from build123d import *

# Parameters (mm, degrees)
F3_W           = 38.1
F3_H           = 32.95
F3_W_2         = 34.5
F3_H_2         = 29.35
F4_DEPTH       = 102
F6_W           = 5.6
F6_H           = 6
F7_DEPTH       = 1.8
F5_R           = 1.5
F9_DEPTH       = 2
F10_DEPTH      = 32.951
F10_DEPTH_BACK = 25
F11_W          = 38.1
F11_H          = 34.95
F12_DEPTH      = 1.8
F14_DEPTH      = 3.8
F15_R          = 2.7
F16_DEPTH      = 2
F16_DEPTH_BACK = 31.151
F17_DEPTH      = 31.15
F19_DEPTH      = 25
F20_R          = 2.5
F21_R          = 2
F24_DEPTH      = 28
F25_R          = 0.89999


# Not quite as in the source:
# - a fillet or chamfer is up to 0.001 mm smaller than in the source, because OpenCascade refuses the exact size


with BuildPart() as f4:
    # F3 (on Top) → F4 (new body)
    with BuildSketch(Plane.XY):
        Rectangle(F3_W, F3_H)
        Rectangle(F3_W_2, F3_H_2, mode=Mode.SUBTRACT)
    extrude(amount=F4_DEPTH)


with BuildPart() as f7:
    # F6 (on face) → F7 (new body)
    with BuildSketch(Plane.XZ.offset(16.475)):
        with Locations((-16.25, 105)):
            Rectangle(F6_W, F6_H)
    extrude(amount=-F7_DEPTH)


with BuildPart() as f7b:
    # F6 (on face) → F7, piece 2 (new body)
    with BuildSketch(Plane.XZ.offset(16.475)):
        with Locations((16.25, 105)):
            Rectangle(F6_W, F6_H)
    extrude(amount=-F7_DEPTH)


with BuildPart() as f4_1:
    add(f4.part)

    # F8: union F7, F7b
    add(f7.part)
    add(f7b.part)

    # F5 (on face) + F8_face (on face) → F9 (join)
    with BuildSketch(Plane.XZ.offset(16.475)):
        Polygon((16.25, 102), (-16.2500000167, 102), (-19.05, 102), (-19.05, 0), (19.05, 0), (19.05, 102), align=None)
        with Locations((-16.25, 2)):
            Circle(F5_R, mode=Mode.SUBTRACT)
        with Locations((16.25, 2)):
            Circle(F5_R, mode=Mode.SUBTRACT)
    with BuildSketch(Plane(origin=(0, -16.475, 51.9178934588), x_dir=(1, 0, 0), z_dir=(0, -1, 0))):
        Polygon((-19.05, 56.0821065412), (-19.05, -51.9178934588), (19.05, -51.9178934588), (19.05, 56.0821065412), (13.45, 56.0821065412), (13.45, 50.0821065412), (-13.45, 50.0821065412), (-13.45, 56.0821065412), align=None)
    extrude(amount=F9_DEPTH)

    # F5 (on face) → F10 (cut, two sides)
    with BuildSketch(Plane.XZ.offset(16.475)) as f10_sk:
        with Locations((-16.25, 2)):
            Circle(F5_R)
        with Locations((-16.25, 103.5)):
            Circle(F5_R)
        with Locations((16.25, 103.5)):
            Circle(F5_R)
        with Locations((16.25, 2)):
            Circle(F5_R)
    extrude(amount=-F10_DEPTH, mode=Mode.SUBTRACT)
    extrude(f10_sk.sketch, amount=F10_DEPTH_BACK, mode=Mode.SUBTRACT)

    # F11 (on face) → F12 (join)
    with BuildSketch(Plane(origin=(0, 0, 0), x_dir=(1, 0, 0), z_dir=(0, 0, -1))):
        with Locations((0, 1)):
            Rectangle(F11_W, F11_H)
    extrude(amount=F12_DEPTH)

    # F13 (on face) → F14 (join)
    with BuildSketch(Plane.XZ.offset(18.475)):
        Polygon((-19.05, 100), (-19.05, 108), (-21.1935935394, 108), align=None)
        Polygon((-21.05, -1.8), (-19.05, -1.8), (-19.05, 6.2), align=None)
        Polygon((21.05, -1.8), (19.05, 6.2), (19.05, -1.8), align=None)
        Polygon((21.1935935394, 108), (19.05, 108), (19.05, 100), align=None)
        Polygon((13.45, 102), (13.45, 108), (11.45, 102), align=None)
        Polygon((-13.45, 102), (-11.45, 102), (-13.45, 108), align=None)
    extrude(amount=-F14_DEPTH)

    # F15 (on face) → F16 (cut, two sides)
    with BuildSketch(Plane(origin=(0, -14.675, 0), x_dir=(-1, 0, 0), z_dir=(0, 1, 0))) as f16_sk:
        with Locations((-16.25, 103.5)):
            Circle(F15_R)
        with Locations((16.25, 103.5)):
            Circle(F15_R)
        with Locations((-16.25, 2)):
            Circle(F15_R)
        with Locations((16.25, 2)):
            Circle(F15_R)
    extrude(amount=-F16_DEPTH, mode=Mode.SUBTRACT)
    extrude(f16_sk.sketch, amount=F16_DEPTH_BACK, mode=Mode.SUBTRACT)

    # F17 (add, through all): faces of the model
    f17_faces = [f4_1.faces().sort_by_distance(p)[0] for p in [
        (-19.7166666667, -14.675, 0.8666666667),
        (19.7166666667, -14.675, 0.8666666667),
    ]]
    extrude(f17_faces, amount=F17_DEPTH)

    # F18 (on face) → F19 (cut)
    with BuildSketch(Plane(origin=(0, 0, -1.8), x_dir=(1, 0, 0), z_dir=(0, 0, -1))):
        with BuildLine():
            Line((10, 9.9949482828), (0, 9.9949482828))
            Line((0, 9.9949482828), (0, 0))
            Line((0, 0), (15, 0))
            Line((15, 0), (15, 4.9949482828))
            ThreePointArc((15, 4.9949482828), (13.5355339059, 8.5304821888), (10, 9.9949482828))
        make_face()
        with BuildLine():
            Line((0, 0), (0, 9.9949482828))
            Line((0, 9.9949482828), (-10, 9.9949482828))
            ThreePointArc((-10, 9.9949482828), (-13.5355339059, 8.5304821888), (-15, 4.9949482828))
            Line((-15, 4.9949482828), (-15, 0))
            Line((-15, 0), (0, 0))
        make_face()
        with BuildLine():
            Line((15, 0), (0, 0))
            Line((0, 0), (0, -9.9949482828))
            Line((0, -9.9949482828), (10, -9.9949482828))
            ThreePointArc((10, -9.9949482828), (13.5355339059, -8.5304821888), (15, -4.9949482828))
            Line((15, -4.9949482828), (15, 0))
        make_face()
        with BuildLine():
            Line((0, -9.9949482828), (0, 0))
            Line((0, 0), (-15, 0))
            Line((-15, 0), (-15, -4.9949482828))
            ThreePointArc((-15, -4.9949482828), (-13.5355339059, -8.5304821888), (-10, -9.9949482828))
            Line((-10, -9.9949482828), (0, -9.9949482828))
        make_face()
    extrude(amount=-F19_DEPTH, mode=Mode.SUBTRACT)

    # F20
    f20_edges = [f4_1.edges().sort_by_distance(p)[0] for p in [
        (-19.05, 16.475, 54.1),
        (19.05, 16.475, 54.1),
        (19.05, -18.475, 53.1),
        (-19.05, -18.475, 53.1),
    ]]
    fillet(f20_edges, radius=F20_R)

    # F21
    f21_edges = [f4_1.edges().sort_by_distance(p)[0] for p in [
        (-13.45, -16.575, 108),
        (-21.193594, -16.575, 108),
        (13.45, -16.575, 108),
        (21.193594, -16.575, 108),
    ]]
    fillet(f21_edges, radius=F21_R)

    # F23 (on face) → F24 (join)
    with BuildSketch(Plane.YZ.offset(14.0050055679)):
        Polygon((14.5708874184, 101.9686584017), (16.475, 102), (14.7648992834, 106.6984631039), (12.8493792929, 106.6984631039), align=None)
    extrude(amount=-F24_DEPTH)

    # F25 (radius 0.9 in the source; OpenCascade refuses exactly that, so slightly less here)
    f25_edges = [f4_1.edges().sort_by_distance(p)[0] for p in [
        (0.005006, 14.764899, 106.698463),
        (0.005006, 12.849379, 106.698463),
    ]]
    fillet(f25_edges, radius=F25_R)


solid = f4_1.part
Build history of the part. All positions in model axes, mm. A direction names the side the tool comes from. Give positions to 0.01 mm unless a question says otherwise; leave off trailing zeros. Order: outer loops, then holes, each group sorted by start corner. A loop starts at its lowest first (then second) coordinate and runs counter-clockwise, first axis right, second up. Notation, with made-up numbers: M 25.5,73 L 32.5,73 A25 ccw 32.5,94 Z; hole C -22.5,40 d2. An arc over 180 degrees is marked long. Use one line per item in the form item = value.
Q1. Pin check, flat tips, straight feed: P1, Ø0.7, axis at y = -0.5, z = -1, coming from the +X side; P2, Ø15, axis at y = -2, z = 30.5, coming from the -X side; P3, Ø3.5, axis at y = 15.5, z = 105, coming from the -X side (3 decimals). Stop position of each tip, or through.
Conclusion:
P1 = 20.94
P2 = -19.05
P3 = -13.995
Q2. Wall check: probe 1 along Z at (x, y) = (16.25, -17.15); probe 2 along X at (y, z) = (7, 59). Give the ranges that are in metal, low to high.
Conclusion:
probe_1 = -1.8 to 0.5, 3.5 to 102, 105 to 108
probe_2 = -19.05 to -17.25, 17.25 to 19.05
Q3. Which spindle directions (+Z, -Z, +X, -X, +Y, -Y) get a long thin tool onto all of the face, cutting with end or side? Do faces 1 (the flat face through (0, -17, 102)), 2 (the cylindrical face through (18.3, 15.76, 53.43)), 3 (the flat face through (-17.4, -16.675, 0.8)), 4 (the cylindrical face through (-13.496, -8.569, -0.913)). Say none if no direction does.
Conclusion:
face_1 = +Z, -Y
face_2 = +Z, +X, +Y
face_3 = +Y
face_4 = +Z, -Z
Q4. Pull direction X, two halves, no side cores. Call faces 5 (the flat face through (15.1, -16.675, 0.8)), 6 (the flat face through (0.2, 15.74, 104.02)), 7 (the flat face through (0, -12, 0)), 8 (the cylindrical face through (20.189, -16.548, 107.197)): released by +X, released by -X, zero draft, split by the parting line, or undercut.
Conclusion:
face_5 = undercut
face_6 = zero draft
face_7 = undercut
face_8 = released by +X
Q5. Slice it at D-D, the plane y = -9. Write the cut outline in (x, z) (3 decimals).
Conclusion:
outline = M -21.05,-1.8 L -12.993,-1.8 L -12.993,0 L -14.436,0 A2.7 cw long -17.25,4.508 L -17.25,100.992 A2.7 cw -18.495,102 L -19.05,102 L -19.05,6.2 Z; M 12.993,-1.8 L 21.05,-1.8 L 19.05,6.2 L 19.05,102 L 18.495,102 A2.7 cw 17.25,100.992 L 17.25,4.508 A2.7 cw long 14.436,0 L 12.993,0 Z
Q6. Slice it at C-C, the plane z = 42. Write the cut outline in (x, y) (3 decimals), and give its area (3 significant figures).
Conclusion:
outline = M -19.05,-15.975 A2.5 ccw -16.55,-18.475 L 16.55,-18.475 A2.5 ccw 19.05,-15.975 L 19.05,13.975 A2.5 ccw 16.55,16.475 L -16.55,16.475 A2.5 ccw -19.05,13.975 Z; hole M -17.25,-14.675 L 17.25,-14.675 L 17.25,14.675 L -17.25,14.675 Z
area = 314 mm2
Q7. Slice it at A-A, the plane z = 2. Write the cut outline in (x, y) (3 decimals), and give its area (3 significant figures).
Conclusion:
outline = M -20.1,-18.475 L -17.75,-18.475 L -17.75,-16.675 L -18.95,-16.675 L -18.95,16.475 L -20.1,16.475 Z; M -14.75,-18.475 L 14.75,-18.475 L 14.75,-16.675 L 13.55,-16.675 L 13.55,-14.675 L -13.55,-14.675 L -13.55,-16.675 L -14.75,-16.675 Z; M -13.55,14.675 L 13.55,14.675 L 13.55,16.475 L -13.55,16.475 Z; M 17.75,-18.475 L 20.1,-18.475 L 20.1,16.475 L 18.95,16.475 L 18.95,-16.675 L 17.75,-16.675 Z
area = 241 mm2
